Geometry check sheet. Reference: the model listing, model coordinates, mm. A direction names the side the tool comes from. Round coordinates to 2 decimals unless told otherwise and drop trailing zeros. Order: outer loops, then holes, each group sorted by start corner. A loop starts at its lowest first (then second) coordinate and runs counter-clockwise, first axis right, second up. Notation, with made-up numbers: (22, 12.25) - (49, 12.25) arc R27 cw to (49, 36.25) - close; hole circle Ø7 at (-39.5, -0.5). An arc over 180 degrees is marked (long way). One line per question, with ' | ' between items. Start each with the question number.
Q1. Gauge pin test, flat end, axial feed: P1, Ø2, axis at y = 5.5, z = 11, coming from the +X side. Record the tip position at first contact, or that the pin passes through.
Q2. Sectioned sample at B-B, the plane x = -340. Enter the section's corners in (y, z).
Q3. Sectioned sample at C-C, the plane z = 8.5. Give the number of separate pieces and of enclosed holes in the cut face, then the cut area to 3 significant figures.
Q4. Tool access check on faces 5 (the face through (-333.384, -9, 13)), 6 (the face through (-388.06, 15.53, 12.52)), 7 (the face through (-358, -11.621, 13)). Record the directions out of +Z, -Z, +X, -X, +Y, -Y that give a thin tool (end or side, any length) a straight path to the whole face; none if there is none.
Q5. Sectioned sample at A-A, the plane x = -355.5. Enter the section's corners in (y, z), then the cut area to 3 significant figures.
Q6. Mould release check, pull along Y, two halves, no side actions. Record for faces 1 (the face through (-321, 1.379, 13)), 2 (the face through (-366.5, 21.8, 0)), 3 (the face through (-395.905, -10.1, 12.522)), 4 (the face through (-332, 23.879, 13)): +Y half, -Y half, draft (parallel to the pull), parting line (faces both ways), or undercut.
Q7. Material ranges on line 1 along Y through (x, z) = (-391.5, 20.25); line 2 along X through (y, z) = (23.5, 7); line 3 along Y through (x, z) = (-363, 9.75), recorded low to high.
```python
from build123d import *

# Parameters (mm, degrees)
SKETCH1_R      = 3.4
EXTRUDE1_DEPTH = 25.4


with BuildPart() as part:
    # Sketch1 → Extrude1 (new body)
    with BuildSketch(Plane.XY):
        Polygon((-367.383665724, -5.145535609), (-367.383665724, -8.620535609), (-370.383665724, -8.620535609), (-370.383665724, -7.120535609), (-373.383665724, -7.120535609), (-373.383665724, -11.620535609), (-341.383665724, -11.620535609), (-341.383665724, -7.120535609), (-344.383665724, -7.120535609), (-344.383665724, -8.620535609), (-347.383665724, -8.620535609), (-347.383665724, -5.145535609), (-341.608665724, 0.629464391), (-333.158665724, 0.629464391), (-327.383665724, -5.145535609), (-327.383665724, -8.620535609), (-330.383665724, -8.620535609), (-330.383665724, -7.120535609), (-333.383665724, -7.120535609), (-333.383665724, -11.620535609), (-320.383665724, -11.620535609), (-317.383665724, -8.620535609), (-317.383665724, 4.315964391), (-321.883665724, 4.315964391), (-321.883665724, 1.379464391), (-320.383665724, 1.379464391), (-320.383665724, -1.912635609), (-323.566565724, -1.912635609), (-329.633665724, 4.154464391), (-329.633665724, 12.604464391), (-323.566565724, 18.671564391), (-320.383665724, 18.671564391), (-320.383665724, 15.379464391), (-321.883665724, 15.379464391), (-321.883665724, 12.442964391), (-317.383665724, 12.442964391), (-317.383665724, 25.379464391), (-320.383665724, 28.379464391), (-333.383665724, 28.379464391), (-333.383665724, 23.879464391), (-330.383665724, 23.879464391), (-330.383665724, 25.379464391), (-327.383665724, 25.379464391), (-327.383665724, 21.904464391), (-333.158665724, 16.129464391), (-341.608665724, 16.129464391), (-347.383665724, 21.904464391), (-347.383665724, 25.379464391), (-344.383665724, 25.379464391), (-344.383665724, 23.879464391), (-341.383665724, 23.879464391), (-341.383665724, 28.379464391), (-373.383665724, 28.379464391), (-373.383665724, 23.879464391), (-370.383665724, 23.879464391), (-370.383665724, 25.379464391), (-367.383665724, 25.379464391), (-367.383665724, 21.904464391), (-373.158665724, 16.129464391), (-381.608665724, 16.129464391), (-387.383665724, 21.904464391), (-387.383665724, 25.379464391), (-384.383665724, 25.379464391), (-384.383665724, 23.879464391), (-381.383665724, 23.879464391), (-381.383665724, 28.379464391), (-394.383665724, 28.379464391), (-397.383665724, 25.379464391), (-397.383665724, 12.379464391), (-392.883665724, 12.379464391), (-392.883665724, 15.379464391), (-394.383665724, 15.379464391), (-394.383665724, 18.379464391), (-390.908665724, 18.379464391), (-385.133665724, 12.604464391), (-385.133665724, 4.154464391), (-390.908665724, -1.620535609), (-394.383665724, -1.620535609), (-394.383665724, 1.379464391), (-392.883665724, 1.379464391), (-392.883665724, 4.379464391), (-397.383665724, 4.379464391), (-397.383665724, -8.620535609), (-394.383665724, -11.620535609), (-381.383665724, -11.620535609), (-381.383665724, -7.120535609), (-384.383665724, -7.120535609), (-384.383665724, -8.620535609), (-387.383665724, -8.620535609), (-387.383665724, -5.145535609), (-381.608665724, 0.629464391), (-373.158665724, 0.629464391), align=None)
        with Locations((-337.383665724, 8.379464391)):
            Circle(SKETCH1_R, mode=Mode.SUBTRACT)
        with Locations((-377.383665724, 8.379464391)):
            Circle(SKETCH1_R, mode=Mode.SUBTRACT)
        Polygon((-373.130411724, 11.469634391), (-372.126354724, 8.379464391), (-373.130411724, 5.289294391), (-375.759067724, 3.379464391), (-375.883665724, 3.379464391), (-375.883665724, 2.129464391), (-372.537345724, 2.129464391), (-365.883665724, -4.524215609), (-365.883665724, -9.620535609), (-348.883665724, -9.620535609), (-348.883665724, -4.524215609), (-342.229985724, 2.129464391), (-338.883665724, 2.129464391), (-338.883665724, 3.379464391), (-339.008263724, 3.379464391), (-341.636919724, 5.289294391), (-342.640976724, 8.379464391), (-341.636919724, 11.469634391), (-339.008263724, 13.379464391), (-338.883665724, 13.379464391), (-338.883665724, 14.629464391), (-342.229985724, 14.629464391), (-348.883665724, 21.283144391), (-348.883665724, 26.379464391), (-365.883665724, 26.379464391), (-365.883665724, 21.283144391), (-372.537345724, 14.629464391), (-375.883665724, 14.629464391), (-375.883665724, 13.379464391), (-375.759067724, 13.379464391), align=None, mode=Mode.SUBTRACT)
        Polygon((-382.126432724, 14.879464391), (-386.581320724, 19.334352391), (-388.338553724, 17.577119391), (-383.883665724, 13.122231391), (-383.883665724, 10.379464391), (-382.129453724, 10.379464391), (-379.383665724, 13.125252391), (-379.383665724, 14.879464391), align=None, mode=Mode.SUBTRACT)
        Polygon((-332.640898724, 1.879464391), (-328.186010724, -2.575423609), (-326.428777724, -0.818190609), (-330.883665724, 3.636697391), (-330.883665724, 6.379464391), (-332.637877724, 6.379464391), (-335.383665724, 3.633676391), (-335.383665724, 1.879464391), align=None, mode=Mode.SUBTRACT)
        Polygon((-383.883665724, 3.636697391), (-388.338553724, -0.818190609), (-386.581320724, -2.575423609), (-382.126432724, 1.879464391), (-379.383665724, 1.879464391), (-379.383665724, 3.633676391), (-382.129453724, 6.379464391), (-383.883665724, 6.379464391), align=None, mode=Mode.SUBTRACT)
        Polygon((-330.883665724, 13.122231391), (-326.428777724, 17.577119391), (-328.186010724, 19.334352391), (-332.640898724, 14.879464391), (-335.383665724, 14.879464391), (-335.383665724, 13.125252391), (-332.637877724, 10.379464391), (-330.883665724, 10.379464391), align=None, mode=Mode.SUBTRACT)
        Polygon((-393.865898724, 27.129464391), (-396.133665724, 24.861697391), (-396.133665724, 19.629464391), (-388.633665724, 19.629464391), (-388.633665724, 27.129464391), align=None, mode=Mode.SUBTRACT)
        Polygon((-320.901432724, -10.370535609), (-318.633665724, -8.102768609), (-318.633665724, -2.870535609), (-326.133665724, -2.870535609), (-326.133665724, -10.370535609), align=None, mode=Mode.SUBTRACT)
        Polygon((-396.133665724, -2.870535609), (-396.133665724, -8.102768609), (-393.865898724, -10.370535609), (-388.633665724, -10.370535609), (-388.633665724, -2.870535609), align=None, mode=Mode.SUBTRACT)
        Polygon((-318.633665724, 19.629464391), (-318.633665724, 24.861697391), (-320.901432724, 27.129464391), (-326.133665724, 27.129464391), (-326.133665724, 19.629464391), align=None, mode=Mode.SUBTRACT)
    extrude(amount=EXTRUDE1_DEPTH)


solid = part.part
```
Determined:
1) P1: stops at x = -329.63
2) outline: (0.63, 0) - (2.13, 0) - (2.13, 25.4) - (0.63, 25.4) - close; (4.1, 0) - (6.21, 0) - (6.21, 25.4) - (4.1, 25.4) - close; (10.55, 0) - (12.66, 0) - (12.66, 25.4) - (10.55, 25.4) - close; (14.63, 0) - (16.13, 0) - (16.13, 25.4) - (14.63, 25.4) - close
3) separate pieces: 1 | enclosed holes: 11 | area: 871 mm2
4) face 5: +Z, -Z, -Y | face 6: +Z, -Z | face 7: +Z, -Z, +X, -X, -Y
5) outline: (-11.62, 0) - (-9.62, 0) - (-9.62, 25.4) - (-11.62, 25.4) - close; (26.38, 0) - (28.38, 0) - (28.38, 25.4) - (26.38, 25.4) - close | area: 102 mm2
6) face 1: undercut | face 2: draft | face 3: -Y half | face 4: undercut
7) line 1: y = -11.62 to -10.37, -2.87 to -1.62, 18.38 to 19.63, 27.13 to 28.38 | line 2: x = -397.38 to -396.13, -388.63 to -387.38, -367.38 to -365.88, -348.88 to -347.38, -327.38 to -326.13, -318.63 to -317.38 | line 3: y = -11.62 to -9.62, 26.38 to 28.38
